For this review, take the finished solid that the model builds, in its own axes (mm). A direction names the side the tool comes from. Coordinates: 2 decimals unless noted, no trailing zeros. Order: outer loops, then holes, each group sorted by start corner. A loop starts at its lowest first (then second) coordinate and runs counter-clockwise, first axis right, second up. Notation, with made-up numbers: (-33.5, 32.5) -> (3.5, 32.5) arc R13 ccw to (3.5, 46.5) -> close; hole circle Ø1 at (-15, 40). An arc over 180 degrees is marked (long way). Answer as a JSON object with one key per item and string values. Group by question number.
1) Add section A-A, the plane z = 98.5. Write out the cut boundary in (x, y).
2) For pin 1 (8 mm diameter, centred on x = 473, y = -386.5, fed in from -Z); pin 2 (4 mm diameter, centred on y = -866, z = 93.5, fed in from +X); pin 3 (2 mm diameter, centred on x = -172, y = -121.5, fed in from +Z), all flat-tipped, find the tip position at first contact; note any pin that passes through.
3) Add section D-D, the plane x = 508. Write out the cut boundary in (y, z).
4) Machinability: for faces 1 (the cylindrical face through (-204.11, -504.9, 725.33)), 2 (the flat face through (0, -951, 417)), 3 (the flat face through (531.633, -495, -110)), 4 (the cylindrical face through (638.86, -504.9, 795.26)), which of the approach directions +Z, -Z, +X, -X, +Y, -Y give a long, thin tool a straight path to every point of the face, cutting with its end or side? Answer none if there is none.
5) Draft analysis for pull direction X (two halves, no side actions). For faces 5 (the cylindrical face through (567.375, -115.036, 345.269)), 6 (the cylindrical face through (186.53, -45.11, -116.86)), 7 (the cylindrical face through (638.86, -954.89, 345.27)), state which applies: +X half, -X half, draft (parallel to the pull), parting line (faces both ways), or undercut.
6) Add section C-C, the plane y = -270. Write out the cut boundary in (x, z).
7) Wall thickness on L1, parallel to Z at x = 277.5, y = -841; L2, parallel to Y at x = 429.5, z = 111; L3, parallel to X at y = -590, z = 554: over which ranges is each line inside the solid? List them lowest first.
8) Add section B-B, the plane x = 117.5. Write out the cut boundary in (y, z).
from build123d import *

# Parameters (mm, degrees)
F0_W     = 1000
F0_H     = 1000
F1_DEPTH = 1000
F2_R     = 150
F3_W     = 400
F3_H     = 290
F4_DEPTH = 500
F5_T     = 100
F6_W     = 700
F6_H     = 700
F7_DEPTH = 500


# Not quite as in the source:
# - a shell that OpenCascade refuses in one call is made with other operations: the cavity is built on its own and cut out


with BuildPart() as f1:
    # F0 (on Front) → F1 (new body)
    with BuildSketch(Plane.XZ):
        with Locations((181.6326389278, 340.3687052429)):
            Rectangle(F0_W, F0_H)
    extrude(amount=F1_DEPTH)

    # F2
    f2_edges = [f1.edges().sort_by_distance(p)[0] for p in [
        (181.632639, -1000, 840.368705),
        (681.632639, -500, 840.368705),
        (681.632639, -1000, 340.368705),
        (-318.367361, -1000, 340.368705),
        (-318.367361, -500, 840.368705),
        (181.632639, 0, 840.368705),
        (681.632639, 0, 340.368705),
        (-318.367361, 0, 340.368705),
        (181.632639, -1000, -159.631295),
        (681.632639, -500, -159.631295),
        (-318.367361, -500, -159.631295),
        (181.632639, 0, -159.631295),
    ]]
    fillet(f2_edges, radius=F2_R)

    # F3 (on face) → F4 (cut)
    with BuildSketch(Plane.XZ.offset(1000)):
        with Locations((200, 419.5188772678)):
            Rectangle(F3_W, F3_H)
    extrude(amount=-F4_DEPTH, mode=Mode.SUBTRACT)

    # F5: shell of thickness 100, made by hand


with BuildPart() as f5_core1:
    # F5_t2: copy of F1
    add(f1.part)

    # the walls: a layer under each face that stays
    f5_faces = [f5_core1.faces().sort_by_distance(p)[0] for p in [
        (-318.3673610722, -500, 340.3687052429),
        (-274.4333782502, -956.066017178, 340.3687052429),
        (-274.4333782502, -500, 796.4347224209),
        (-274.4333782502, -500, -115.6973119351),
        (-274.4333782502, -43.933982822, 340.3687052429),
        (-274.4333782502, -925, 765.3687052429),
        (-51.7006944055, -1000, 107.0353719095),
        (-243.3673610722, -925, -115.6973119351),
        (-243.3673610722, -43.933982822, 765.3687052429),
        (181.6326389278, -500, 840.3687052429),
        (-243.3673610722, -75, -115.6973119351),
        (181.6326389278, -500, -159.6312947571),
        (181.6326389278, 0, 340.3687052429),
        (181.6326389278, -956.066017178, 796.4347224209),
        (637.6986561058, -956.066017178, 340.3687052429),
        (181.6326389278, -956.066017178, -115.6973119351),
        (200, -750, 564.5188772678),
        (181.6326389278, -43.933982822, 796.4347224209),
        (637.6986561058, -500, 796.4347224209),
        (181.6326389278, -43.933982822, -115.6973119351),
        (637.6986561058, -500, -115.6973119351),
        (637.6986561058, -43.933982822, 340.3687052429),
        (637.6986561058, -925, 765.3687052429),
        (681.6326389278, -500, 340.3687052429),
        (606.6326389278, -925, -115.6973119351),
        (606.6326389278, -43.933982822, 765.3687052429),
        (606.6326389278, -75, -115.6973119351),
    ]]
    thicken(f5_faces, amount=-F5_T, mode=Mode.SUBTRACT)


with BuildPart() as f1_1:
    add(f1.part)

    # what is left inside the walls is the cavity
    f5_cavity = [f5_core1.part.solids().sort_by_distance(p)[0] for p in [
        (181.632639, -101, 223.702039),
    ]]
    add(f5_cavity, mode=Mode.SUBTRACT)

    # F6 (on face) → F7 (cut)
    with BuildSketch(Plane(origin=(0, 0, -159.6312947571), x_dir=(1, 0, 0), z_dir=(0, 0, -1))):
        with Locations((181.6326389278, 500)):
            Rectangle(F6_W, F6_H)
    extrude(amount=-F7_DEPTH, mode=Mode.SUBTRACT)


solid = f1_1.part
Output values:
{
 "1": {"outline": "(-318.37, -850) arc R150 ccw to (-168.37, -1000) -> (531.63, -1000) arc R150 ccw to (681.63, -850) -> (681.63, -150) arc R150 ccw to (531.63, 0) -> (-168.37, 0) arc R150 ccw to (-318.37, -150) -> close; hole (-218.37, -850) arc R50 ccw to (-168.37, -900) -> (531.63, -900) arc R50 ccw to (581.63, -850) -> (581.63, -150) arc R50 ccw to (531.63, -100) -> (-168.37, -100) arc R50 ccw to (-218.37, -150) -> close"},
 "2": {"pin 1": "stops at z = 740.37", "pin 2": "stops at x = 680.98", "pin 3": "stops at z = 837.78"},
 "3": {"outline": "(-1000, -9.63) arc R150 ccw to (-850, -159.63) -> (-850, -59.63) arc R50 cw to (-900, -9.63) -> (-900, 690.37) arc R50 cw to (-850, 740.37) -> (-150, 740.37) arc R50 cw to (-100, 690.37) -> (-100, -9.63) arc R50 cw to (-150, -59.63) -> (-150, -159.63) arc R150 ccw to (0, -9.63) -> (0, 690.37) arc R150 ccw to (-150, 840.37) -> (-850, 840.37) arc R150 ccw to (-1000, 690.37) -> close"},
 "4": {"face 1": "none", "face 2": "-Y", "face 3": "-Z", "face 4": "+Z, +X, +Y, -Y"},
 "5": {"face 5": "undercut", "face 6": "draft", "face 7": "+X half"},
 "6": {"outline": "(-318.37, -9.63) arc R150 ccw to (-168.37, -159.63) -> (-168.37, -59.63) arc R50 cw to (-218.37, -9.63) -> (-218.37, 690.37) arc R50 cw to (-168.37, 740.37) -> (531.63, 740.37) arc R50 cw to (581.63, 690.37) -> (581.63, -9.63) arc R50 cw to (531.63, -59.63) -> (531.63, -159.63) arc R150 ccw to (681.63, -9.63) -> (681.63, 690.37) arc R150 ccw to (531.63, 840.37) -> (-168.37, 840.37) arc R150 ccw to (-318.37, 690.37) -> close"},
 "7": {"L1": "z = 564.52 to 664.52, 740.37 to 840.37", "L2": "y = -1000 to -900, -100 to 0", "L3": "x = -318.37 to -218.37, 581.63 to 681.63"},
 "8": {"outline": "(-1000, -9.63) arc R150 ccw to (-850, -159.63) -> (-850, -59.63) arc R50 cw to (-900, -9.63) -> (-900, 274.52) -> (-1000, 274.52) -> close; (-1000, 564.52) -> (-500, 564.52) -> (-500, 664.52) -> (-900, 664.52) -> (-900, 690.37) arc R50 cw to (-850, 740.37) -> (-150, 740.37) arc R50 cw to (-100, 690.37) -> (-100, -9.63) arc R50 cw to (-150, -59.63) -> (-150, -159.63) arc R150 ccw to (0, -9.63) -> (0, 690.37) arc R150 ccw to (-150, 840.37) -> (-850, 840.37) arc R150 ccw to (-1000, 690.37) -> close"}
}
